The model under review builds one solid part; all positions refer to its coordinate system, in mm. A direction names the side the tool comes from. Coordinates: 2 decimals unless noted, no trailing zeros. Loops run counter-clockwise (first coordinate to the right, second up) from the corner with the lowest first, then second, coordinate; pieces in that order, holes last. Notation, with made-up numbers: (7.5, 3) -> (13.5, 3) arc R20 cw to (13.5, 22) -> close; hole circle Ø3 at (87.5, 36.5). An arc over 180 degrees is marked (long way). One line per question, with ' | ' between items. Start each with the question number.
Autodesk Inventor part; units mm, degrees
ref_plane "YZ Plane" through (0, 0, 0) normal (1, 0, 0) x (0, 1, 0)
ref_plane "XZ Plane" through (0, 0, 0) normal (0, 1, 0) x (-1, 0, 0)
ref_plane "XY Plane" through (0, 0, 0) normal (0, 0, 1) x (1, 0, 0)
sketch "Sketch1" plane through (0, 0, 0) normal (1, 0, 0) x (0, 1, 0)
  line L0 (0, 90) -> (0, 60)
  line L1 (400, 0) -> (400, 40)
  line L2 (6, 90) -> (0, 90)
  line L3 (360, 0) -> (360, -3)
  line L4 (353, -15) -> (375, -15)
  line L5 (380, -10) -> (380, 0)
  line L6 (353, -15) -> (340, -15) construction
  line L7 (340, -15) -> (340, -11) construction
  line L8 (340, -3) -> (360, -3)
  line L9 (0, 0) -> (360, 0)
  line L10 (380, 0) -> (400, 0)
  line L11 (340, -11) -> (353, -15)
  arc A0 (375, -15) -> (380, -10) centre (375, -10) ccw
  line L12 (340, -11) -> (340, -3)
  line L13 (240, 0) -> (240, -3)
  line L14 (220, -3) -> (240, -3)
  line L15 (220, -11) -> (220, -3)
  line L16 (260, -10) -> (260, 0)
  line L17 (233, -15) -> (255, -15)
  line L18 (233, -15) -> (220, -15) construction
  line L19 (220, -15) -> (220, -11) construction
  line L20 (220, -11) -> (233, -15)
  arc A1 (255, -15) -> (260, -10) centre (255, -10) ccw
  line L21 (120, 0) -> (120, -3)
  line L22 (100, -3) -> (120, -3)
  line L23 (100, -11) -> (100, -3)
  line L24 (140, -10) -> (140, 0)
  line L25 (113, -15) -> (135, -15)
  line L26 (113, -15) -> (100, -15) construction
  line L27 (100, -15) -> (100, -11) construction
  line L28 (100, -11) -> (113, -15)
  arc A2 (135, -15) -> (140, -10) centre (135, -10) ccw
  line L29 (240, 0) -> (260, 0)
  line L30 (120, 0) -> (140, 0)
  line L31 (6, 90) -> (6, 60) construction
  line L32 (0, 60) -> (6, 60)
  line L33 (6, 30) -> (0, 30)
  line L34 (0, 60) -> (0, 30) construction
  line L35 (0, 30) -> (0, 0)
  line L36 (6, 30) -> (6, 0) construction
  line L37 (6, 60) -> (6, 30)
  line L38 (400, 40) -> (380, 40)
  line L39 (380, 40) -> (316.8572, 20)
  line L40 (316.8572, 20) -> (116.5169, 20)
  line L41 (48.9774, 55) -> (6, 115.8967)
  arc A3 (48.9774, 55) -> (116.5169, 20) centre (116.5169, 102.6656) ccw
  line L42 (6, 90) -> (6, 115.8967)
  point P0 (24.2764, 90)
  dimension "d0" = 400
  dimension "d2" = 40
  dimension "d3" = 90
  dimension "d7" = 3
  dimension "d8" = 20
  dimension "d9" = 20
  dimension "d10" = 12
  dimension "d11" = 5
  dimension "d14" = 120
  dimension "d19" = 8
  dimension "d20" = 22
  dimension "d21" = 20
  dimension "d22" = 6
  dimension "d23" = 30
  dimension "d24" = 30
extrude "Extrusion1" add sketch "Sketch1" along normal blind 3
sketch "Sketch2" plane through (3, 0, 0) normal (1, 0, 0) x (0, 0, -1)
  line L0 (-52, 16) -> (-36, 16) construction
  line L1 (-30, 0) -> (0, 0)
  line L2 (-30, 390) -> (-10, 390) construction
  line L3 (0, 400) -> (-40, 400)
  line L4 (0, 380) -> (0, 400)
  line L5 (0, 0) -> (0, 120)
  dimension "d25" = 16
  dimension "d26" = 16
  dimension "d27" = 20
  dimension "d28" = 10
  dimension "d29" = 10
  dimension "d30" = 36
hole "Hole1" at (3, 16, 52) at (3, 16, 36) at (3, 390, 30) at (3, 390, 10) direction (-1, 0, 0) diameter 3.2 end through all
properties part number "Camera mounting side"
1) Consider section A-A, the plane y = 198.5. Write out the cut boundary in (x, z), plus the area to 3 significant figures.
2) Insertion check: pin 1 Ø0.9 at (x, y) = (1.5, 228.5) entering from +Z; pin 2 Ø0.9 at (x, y) = (1.5, 43) entering from -Z; pin 3 Ø0.9 at (x, z) = (1.5, -2) entering from -Y. Each pin has a flat end and moves straight along its axis. Give the tip position at first contact, or say it passes through.
3) Consider section B-B, the plane x = 0.5. Give the number of separate pieces and of enclosed holes in the cut face, plus the area to 3 significant figures.
4) Consider section C-C, the plane z = 66. Write out the cut boundary in (x, y).
5) Mouldability with a two-part tool opening along Y and no side actions: class faces 1 (the face through (0, 169, 17)), 2 (the face through (1.48, 348.87, 30.14)), 3 (the face through (1.48, 27.79, 85.02)) as +Y half, -Y half, draft (parallel to the pull), parting line (faces both ways), or undercut.
6) Machinability: for faces 4 (the face through (3, 169, 17)), 5 (the face through (1.48, 78.97, 29.02)), which of the approach directions +Z, -Z, +X, -X, +Y, -Y give a long, thin tool a straight path to every point of the face, cutting with its end or side? Answer none if there is none.
7) Wall thickness on L1, parallel to Z at x = 0.8, y = 390; L2, parallel to Z at x = 0.1, y = 117; L3, parallel to Z at x = 1.35, y = 16: over which ranges is each line inside the solid? List them lowest first.
Filled sheet:
1) outline: (0, 0) -> (3, 0) -> (3, 20) -> (0, 20) -> close | area: 60.0 mm^2
2) pin 1: z = 20 | pin 2: z = 0 | pin 3: y = 120
3) separate pieces: 1 | enclosed holes: 4 | area: 14,300 mm^2
4) outline: (0, 0) -> (3, 0) -> (3, 41.21) -> (0, 41.21) -> close
5) face 1: draft | face 2: undercut | face 3: +Y half
6) face 4: +Z, -Z, +X, +Y, -Y | face 5: +Z, +X, -X
7) L1: 0 to 8.4, 11.6 to 28.4, 31.6 to 40 | L2: -15 to -3, 0 to 20 | L3: 0 to 34.4, 37.6 to 50.4, 53.6 to 101.73
